```python
from build123d import *

# Parameters (mm, degrees)
F_0150_CYLINDER_SKETCH_R    = 2.5
F_0150_CYLINDER_DEPTH       = 1.5
F_0151_FILLET_R             = 0.375
F_0152_EXTRUDE_DEPTH        = 0.835
F_0152_EXTRUDE_ROTATE_ANGLE = 120
F_0155_CYLINDER_SKETCH_R    = 1
F_0155_CYLINDER_DEPTH       = 7.7
F_0156_CONE_ROTATE_ANGLE    = 90


with BuildPart() as part:
    # 0150_cylinder_Sketch → 0150_cylinder (new body)
    with BuildSketch(Plane.XY):
        Circle(F_0150_CYLINDER_SKETCH_R)
    extrude(amount=F_0150_CYLINDER_DEPTH)

    # 0151_fillet
    f_0151_fillet_edges = [part.edges().sort_by_distance(p)[0] for p in [
        (-2.5, 0, 1.5),
    ]]
    fillet(f_0151_fillet_edges, radius=F_0151_FILLET_R)


with BuildPart() as body_2:
    # 0152_extrude_Sketch → 0152_extrude (new body)
    with BuildSketch(Plane.XY):
        Polygon((0, 0), (0.866025404, 0), (1.299038106, 0.75), (0.866025404, 1.5), (0, 1.5), (-0.433012702, 0.75), align=None)
    extrude(amount=F_0152_EXTRUDE_DEPTH)


with BuildPart() as body_2_1:
    # 0152_extrude_Rotate: read off the stored shape, not the designer's step
    # 0152_extrude_Rotate: moved
    add(body_2.part.rotate(Axis((0, 0, 0), (0, 0, 1)), F_0152_EXTRUDE_ROTATE_ANGLE))


with BuildPart() as body_2_2:
    # 0152_extrude_Translate: moved
    add(body_2_1.part.moved(Location((0.866025404, 0, 0.675))))


with BuildPart() as part_1:
    add(part.part)

    # 0154_sub: cut body 2
    add(body_2_2.part, mode=Mode.SUBTRACT)


with BuildPart() as body_2_2_1:
    # 0155_cylinder_Sketch → 0155_cylinder (new body)
    with BuildSketch(Plane.XY):
        with Locations(Location((0, 0, 0), (0, 0, 180))):
            Circle(F_0155_CYLINDER_SKETCH_R)
    extrude(amount=F_0155_CYLINDER_DEPTH)


with BuildPart() as body_2_2_2:
    # 0155_cylinder_Translate: moved
    add(body_2_2_1.part.moved(Location((0, 0, -7.7))))


with BuildPart() as body_3:
    # 0156_cone_Sketch → 0156_cone (revolve)
    with BuildSketch(Plane.XY, mode=Mode.PRIVATE) as f_0156_cone_sk:
        Polygon((0, 0), (1, 0), (0.7, 0.3), (0, 0.3), align=None)
    revolve(f_0156_cone_sk.sketch.rotate(Axis((0, -100, 0), (0, 1, 0)), 90), axis=Axis((0, -100, 0), (0, 1, 0)))


with BuildPart() as body_3_1:
    # 0156_cone_Rotate: moved
    add(body_3.part.rotate(Axis((0, 0, 0), (1, 0, 0)), F_0156_CONE_ROTATE_ANGLE))


with BuildPart() as body_3_2:
    # 0156_cone_Translate: moved
    add(body_3_1.part.moved(Location((0, 0, -8))))


with BuildPart() as body_2_2_3:
    add(body_2_2_2.part)

    # 0158_add: union body 3
    add(body_3_2.part)


with BuildPart() as part_2:
    add(part_1.part)

    # 0159_add: union body 2 2
    add(body_2_2_3.part)


solid = part_2.part
```
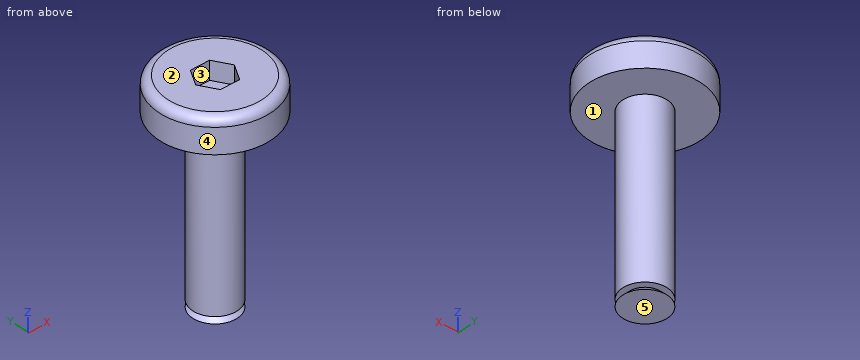
Can you work these out from the model? Positions are in its coordinate system, mm. Face numbers are marked on the shaded views. A direction names the side the tool comes from. Give positions to 0.01 mm unless a question says otherwise; leave off trailing zeros. Order: outer loops, then holes, each group sorted by start corner. A loop starts at its lowest first (then second) coordinate and runs counter-clockwise, first axis right, second up. Notation, with made-up numbers: M 10.5,-37.5 L 33.5,-37.5 A21 cw 33.5,-14.5 Z; hole C 52,73 d4. An arc over 180 degrees is marked long. Write item = value, one per line. Start each with the question number.
Q1. Will this pin go through, and if not, where does the flat tip stop? pin 1 Ø1 at (x, z) = (1, -4.5) entering from -Y.
Q2. We'd pull the mould along Y, two halves only. Please class the marked faces 3, 4 and 5: pulls with the +Y half, pulls with the -Y half, needs draft (parallel to the pull), parting line crosses it, or undercut.
Q3. Suppose I cut it at A-A (x = 0). Write out the boundary of the cut face in (y, z) (3 decimals).
Q4. For the marked faces 1 and 2, which set-ups out of +Z, -Z, +X, -X, +Y, -Y let a thin tool reach every point of the face, with its end or its side?
Q5. I need wall thicknesses on probe 1 along Z at (x, y) = (1.55, -0.15); probe 2 along X at (y, z) = (0.9, -1.75); probe 3 along X at (y, z) = (0.7, -6.75). Which ranges of each line are inside material? Lowest first, please. Write a range as [from, to].
Q6. Suppose I cut it at B-B (z = -6). Write out the boundary of the cut face in (x, y), plus the area to 3 significant figures.
Check result:
q1.pin_1 = -0.87
q2.face_3 = undercut
q2.face_4 = parting line crosses it
q2.face_5 = needs draft
q3.outline = M -2.5,0 L -1,0 L -1,-7.7 L -0.7,-7.7 L -1,-8 L 1,-8 L 0.7,-7.7 L 1,-7.7 L 1,0 L 2.5,0 L 2.5,1.125 A0.375 ccw 2.125,1.5 L 0.75,1.5 L 0.75,0.675 L -0.75,0.675 L -0.75,1.5 L -2.125,1.5 A0.375 ccw -2.5,1.125 Z
q4.face_1 = -Z
q4.face_2 = +Z, +X, -X, +Y, -Y
q5.probe_1 = [0, 1.5]
q5.probe_2 = [-0.44, 0.44]
q5.probe_3 = [-0.71, 0.71]
q6.outline = C 0,0 d2
q6.area = 3.14 mm2
